Part print with two shaded views. Sizes in mm from the minimum x, y, z corner. Give positions to 0.01 mm unless a question says otherwise; leave off trailing zeros. Order: outer loops, then holes, each group sorted by start corner. A loop starts at its lowest first (then second) coordinate and runs counter-clockwise, first axis right, second up. Notation, with made-up numbers: M 71.5,-2.5 L 114.5,-2.5 A20 ccw 114.5,34.5 Z; hole C -39.75,-7.75 d1. An arc over 180 degrees is marked long. Return JSON: item names as keys, results as strings.
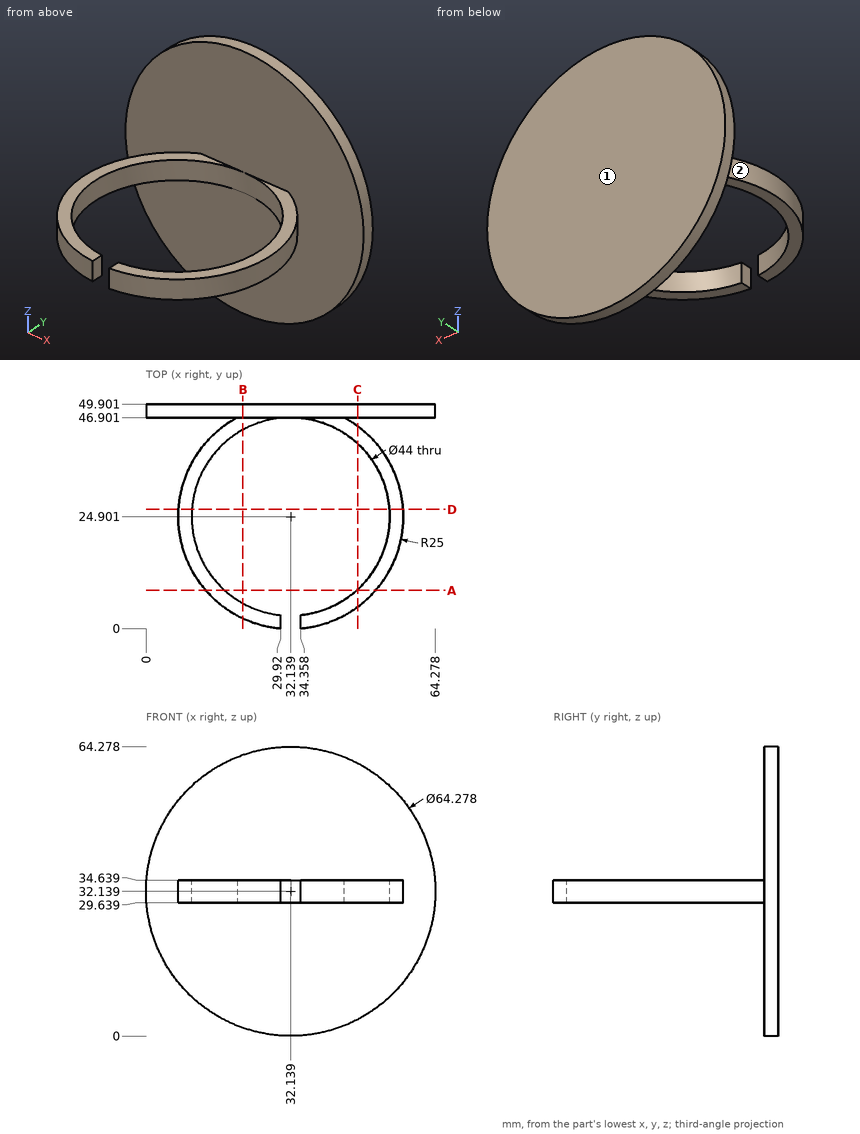
Q1. Band-saw the part on C-C (x = 47). Give the cut face in (y, z) (1 decimal), then the cut area to 3 significant figures.
Established:
{"outline": "M 4.8,29.6 L 8.7,29.6 L 8.7,34.6 L 4.8,34.6 Z; M 41.1,29.6 L 45,29.6 L 45,34.6 L 41.1,34.6 Z; M 46.9,3.6 L 49.9,3.6 L 49.9,60.6 L 46.9,60.6 Z", "area": "210 mm²"}
Q2. Pin check, flat tips, straight feed: pin 1 (5 mm diameter, centred on x = 16.5, y = 14.5, fed in from +Z); pin 2 (5 mm diameter, centred on x = 17, z = 13.5, fed in from -Y); pin 3 (2.5 mm diameter, centred on y = 1, z = 32.5, fed in from +X); pin 4 (2.5 mm diameter, centred on y = 2, z = 31, fed in from -X). Stop position of each tip, or through.
Established:
{"pin 1": "passes through", "pin 2": "stops at y = 46.9", "pin 3": "stops at x = 42.72", "pin 4": "stops at x = 19.64"}
Q3. Two-plate mould, pull along Y, no slides. Class the marked faces 1 and 2: +Y half, -Y half, draft (parallel to the pull), parting line (faces both ways), or undercut.
Established:
{"face 1": "+Y half", "face 2": "undercut"}
Q4. Probe line 1 along Y through (x, z) = (51, 42); line 2 along Z through (x, y) = (9.5, 32.5); line 3 along Y through (x, z) = (54.5, 31). List the from-to ranges inside material, lowest first.
Established:
{"line 1": "y = 46.9 to 49.9", "line 2": "z = 29.64 to 34.64", "line 3": "y = 13.72 to 36.08, 46.9 to 49.9"}
Q5. Band-saw the part on B-B (x = 21.5). Give the cut face in (y, z) (1 decimal).
Established:
{"outline": "M 2.3,29.6 L 5.6,29.6 L 5.6,34.6 L 2.3,34.6 Z; M 44.2,29.6 L 46.9,29.6 L 46.9,1.8 L 49.9,1.8 L 49.9,62.5 L 46.9,62.5 L 46.9,34.6 L 44.2,34.6 Z"}
Q6. Band-saw the part on D-D (y = 26.5). Give the cut face in (x, z).
Established:
{"outline": "M 7.19,29.64 L 10.2,29.64 L 10.2,34.64 L 7.19,34.64 Z; M 54.08,29.64 L 57.09,29.64 L 57.09,34.64 L 54.08,34.64 Z"}
Q7. Band-saw the part on A-A (y = 8.5). Give the cut face in (x, z).
Established:
{"outline": "M 13.27,29.64 L 17.48,29.64 L 17.48,34.64 L 13.27,34.64 Z; M 46.8,29.64 L 51.01,29.64 L 51.01,34.64 L 46.8,34.64 Z"}
